For this review, take the finished solid that the model builds, in its own axes (mm). Face numbers are marked on the shaded views. A direction names the side the tool comes from. Round coordinates to 2 decimals unless told otherwise and drop trailing zeros. Loops run counter-clockwise (first coordinate to the right, second up) from the corner with the lowest first, then second, coordinate; pieces in that order, holes last.
1) Take a section at B-B (y = 6.5). State the section outline as (x, z) points, then the cut area to 3 significant figures.
2) Tool access review of the marked faces 1, 2, 3, 4 and 5: name each direction out of +Z, -Z, +X, -X, +Y, -Y from which nothing blocks a thin tool from reaching the whole face with its end or side.
3) Take a section at D-D (x = 58.5). State the section outline as (y, z) points.
4) Take a section at A-A (z = 2). State the section outline as (x, y) points, then the cut area to 3 significant figures.
5) Mouldability with a two-part tool opening along X and no side actions: class the marked faces 6, 7, 8 and 9 as pulls with the +X half, pulls with the -X half, needs draft (parallel to the pull), parting line crosses it, or undercut.
6) Wall thickness on L1, parallel to X at y = 7, z = 5.25; L2, parallel to X at y = 7.5, z = 7.25; L3, parallel to Z at x = 77.25, y = 9: over which ranges is each line inside the solid? List them lowest first.
7) Take a section at C-C (x = 69.75). State the section outline as (y, z) points.
8) Insertion check: pin 1 (4.5 mm diameter, centred on x = 73, z = 1, fed in from -Y); pin 2 (3 mm diameter, centred on x = 74.979, y = 6.5, fed in from +Z); pin 3 (3 mm diameter, centred on x = 71, y = 17, fed in from -Z); pin 4 (2 mm diameter, centred on x = 70.5, z = 2.5, fed in from +Y). Each pin has a flat end and moves straight along its axis. Give the tip position at first contact, or say it passes through.
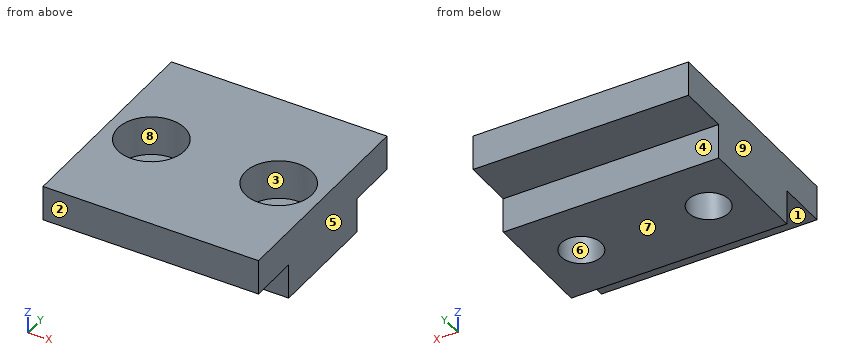
```python
from build123d import *

# Parameters (mm, degrees)
SKETCH1_W           = 24.542
SKETCH1_H           = 13
BOSS_EXTRUDE1_DEPTH = 4
SKETCH2_W           = 24.542
SKETCH2_H           = 24.542
BOSS_EXTRUDE2_DEPTH = 4
SKETCH3_R           = 2.3
CUT_EXTRUDE1_DEPTH  = 9
SKETCH4_R           = 3.8
CUT_EXTRUDE2_DEPTH  = 4.5


with BuildPart() as part:
    # Sketch1 → Boss-Extrude1 (new body)
    with BuildSketch(Plane.XY):
        with Locations((67.729, 6.5)):
            Rectangle(SKETCH1_W, SKETCH1_H)
    extrude(amount=BOSS_EXTRUDE1_DEPTH)

    # Sketch2 → Boss-Extrude2 (add)
    with BuildSketch(Plane.XY.offset(4)):
        with Locations((67.729, 6.5)):
            Rectangle(SKETCH2_W, SKETCH2_H)
    extrude(amount=BOSS_EXTRUDE2_DEPTH)

    # Sketch3 → Cut-Extrude1 (cut, through all)
    with BuildSketch(Plane(origin=(0, 0, 0), x_dir=(-1, 0, 0), z_dir=(0, 0, -1))):
        with Locations((-60.479, 6.5)):
            Circle(SKETCH3_R)
        with Locations((-74.979, 6.5)):
            Circle(SKETCH3_R)
    extrude(amount=-CUT_EXTRUDE1_DEPTH, mode=Mode.SUBTRACT)

    # Sketch4 → Cut-Extrude2 (cut)
    with BuildSketch(Plane.XY.offset(8)):
        with Locations((60.479, 6.5)):
            Circle(SKETCH4_R)
        with Locations((74.979, 6.5)):
            Circle(SKETCH4_R)
    extrude(amount=-CUT_EXTRUDE2_DEPTH, mode=Mode.SUBTRACT)


solid = part.part
```
Response:
1. outline: (55.46, 0) - (58.18, 0) - (58.18, 3.5) - (56.68, 3.5) - (56.68, 8) - (55.46, 8) - close; (62.78, 0) - (72.68, 0) - (72.68, 3.5) - (71.18, 3.5) - (71.18, 8) - (64.28, 8) - (64.28, 3.5) - (62.78, 3.5) - close; (77.28, 0) - (80, 0) - (80, 8) - (78.78, 8) - (78.78, 3.5) - (77.28, 3.5) - close
1. area: 95.7 mm2
2. face 1: -Z, +X, -X, -Y
2. face 2: +Z, -Z, +X, -X, -Y
2. face 3: +Z
2. face 4: -Z, +X, -X, +Y
2. face 5: +Z, -Z, +X, +Y, -Y
3. outline: (-5.77, 4) - (0, 4) - (0, 0) - (5.33, 0) - (5.33, 3.5) - (3.26, 3.5) - (3.26, 8) - (-5.77, 8) - close; (7.67, 0) - (13, 0) - (13, 4) - (18.77, 4) - (18.77, 8) - (9.74, 8) - (9.74, 3.5) - (7.67, 3.5) - close
4. outline: (55.46, 0) - (80, 0) - (80, 13) - (55.46, 13) - close; hole circle Ø4.6 at (60.48, 6.5); hole circle Ø4.6 at (74.98, 6.5)
4. area: 286 mm2
5. face 6: undercut
5. face 7: needs draft
5. face 8: undercut
5. face 9: pulls with the -X half
6. L1: x = 55.46 to 56.71, 64.25 to 71.21, 78.75 to 80
6. L2: x = 55.46 to 56.81, 64.15 to 71.31, 78.65 to 80
6. L3: z = 0 to 3.5
7. outline: (-5.77, 4) - (0, 4) - (0, 0) - (13, 0) - (13, 4) - (18.77, 4) - (18.77, 8) - (-5.77, 8) - close
8. pin 1: stops at y = 0
8. pin 2: passes through
8. pin 3: stops at z = 4
8. pin 4: stops at y = 13
